The figure shows three views and two pictorial views of one solid part (mm, origin at its lowest corner). Answer the questions. A direction names the side the tool comes from. Coordinates: 2 decimals unless noted, no trailing zeros. Order: outer loops, then holes, each group sorted by start corner. A loop starts at its lowest first (then second) coordinate and runs counter-clockwise, first axis right, second up. Notation, with made-up numbers: M -31.75,62 L 15.25,62 A28 cw 15.25,99 Z; hole C 83,14.5 d6. An arc over 180 degrees is marked long. Write item = value, one per line. Start each with the question number.
Q1. Determine the mould class of the marked faces 1, 2 and 3 for opening direction Y: released by +Y, released by -Y, zero draft, split by the parting line, or undercut.
Q2. Each of these flat-tipped pins is pushed along its axis until it touches: P1, Ø4, axis at x = 20, z = 9, coming from the -Y side; P2, Ø9.5, axis at x = 41, y = 25.5, coming from the +Z side. Where does it stop, or does it pass through?
Q3. A tool of negligible diameter and unlimited length cuts with its end or side. For the marked faces 4 and 5, from which of +Z, -Z, +X, -X, +Y, -Y can it reach the whole face along a straight path? Write none if from no direction.
Q4. Find section A-A on y = 28. Give the vertices of the cut face in (x, z).
Q5. Straight lines are drawn through the part: line 1 along Y through (x, z) = (87.5, 6) (1 decimal); line 2 along Y through (x, z) = (9, 6.75) (1 decimal); line 3 along X through (y, z) = (16.5, 8.75). For each, find the intervals that lie inside material, in ascending order.
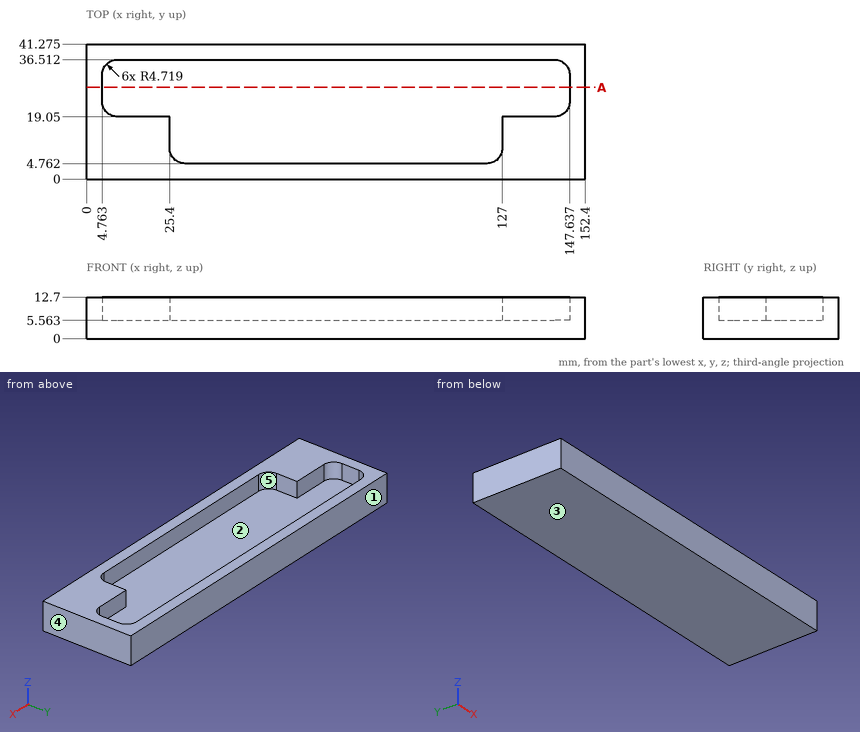
Findings below:
q1.face_1 = released by +Y
q1.face_2 = undercut
q1.face_3 = zero draft
q2.P1 = 0
q2.P2 = 5.56
q3.face_4 = +Z, -Z, +X, +Y, -Y
q3.face_5 = +Z
q4.outline = M 0,0 L 152.4,0 L 152.4,12.7 L 147.64,12.7 L 147.64,5.56 L 4.76,5.56 L 4.76,12.7 L 0,12.7 Z
q5.line_1 = 0 to 4.8, 36.5 to 41.3
q5.line_2 = 0 to 19.1, 36.5 to 41.3
q5.line_3 = 0 to 25.4, 127 to 152.4
